Read the model definition and answer for the solid it produces. Units are mm, in the model's axes. A direction names the side the tool comes from. Coordinates: 2 decimals unless noted, no trailing zeros. Write each loop counter-clockwise with the first axis right and the second up, starting at its lowest first coordinate (ties: lowest second). Pieces come first, ordered by that corner, then holes. Notation, with made-up numbers: M 42,-27.5 L 75,-27.5 A17 cw 75,-22.5 Z; hole C -3.75,-11 d7. An arc over 180 degrees is marked long. Write item = value, one per line.
from build123d import *

# Parameters (mm, degrees)
SKETCH_1_W      = 40
SKETCH_1_H      = 53.5
SKETCH_1_R      = 6.25
SKETCH_1_R_2    = 2
SKETCH_1_W_2    = 3.5
SKETCH_1_H_2    = 1.5
SKETCH_1_W_3    = 1.5
SKETCH_1_H_3    = 3.5
EXTRUDE_1_DEPTH = 5
FILLET_1_R      = 3


with BuildPart() as part:
    # ｽｹｯﾁ1 → ﾎﾞｽ - 押し出し1 (new body)
    with BuildSketch(Plane.XY):
        with Locations((20, 26.75)):
            Rectangle(SKETCH_1_W, SKETCH_1_H)
        with Locations((20, 26.75)):
            Circle(SKETCH_1_R, mode=Mode.SUBTRACT)
        with Locations((35, 5)):
            Circle(SKETCH_1_R_2, mode=Mode.SUBTRACT)
        with Locations(Location((5, 5, 0), (0, 0, 180))):
            Circle(SKETCH_1_R_2, mode=Mode.SUBTRACT)
        with Locations((20, 35.75)):
            Rectangle(SKETCH_1_W_2, SKETCH_1_H_2, mode=Mode.SUBTRACT)
        with Locations((11, 26.75)):
            Rectangle(SKETCH_1_W_3, SKETCH_1_H_3, mode=Mode.SUBTRACT)
    extrude(amount=EXTRUDE_1_DEPTH)

    # ﾌｨﾚｯﾄ1
    fillet_1_edges = [part.edges().sort_by_distance(p)[0] for p in [
        (0, 53.5, 2.5),
        (40, 53.5, 2.5),
        (40, 0, 2.5),
        (0, 0, 2.5),
    ]]
    fillet(fillet_1_edges, radius=FILLET_1_R)


solid = part.part
Item 1: Find section A-A (x = 35). Determine the outline of the cut face in (y, z), and give its area (4 significant figures).
Worked answers:
outline = M 0,0 L 3,0 L 3,5 L 0,5 Z; M 7,0 L 53.5,0 L 53.5,5 L 7,5 Z
area = 247.5 mm²
Item 2: Find section B-B (y = 5). Determine the outline of the cut face in (x, z).
Worked answers:
outline = M 0,0 L 3,0 L 3,5 L 0,5 Z; M 7,0 L 33,0 L 33,5 L 7,5 Z; M 37,0 L 40,0 L 40,5 L 37,5 Z
Item 3: Find section D-D (z = 3.4). Determine the outline of the cut face in (x, y), and give its area (3 significant figures).
Worked answers:
outline = M 0,3 A3 ccw 3,0 L 37,0 A3 ccw 40,3 L 40,50.5 A3 ccw 37,53.5 L 3,53.5 A3 ccw 0,50.5 Z; hole C 5,5 d4; hole M 10.25,25 L 11.75,25 L 11.75,28.5 L 10.25,28.5 Z; hole C 20,26.75 d12.5; hole M 18.25,35 L 21.75,35 L 21.75,36.5 L 18.25,36.5 Z; hole C 35,5 d4
area = 1,970 mm²
Item 4: Consider line 1 along Y through (x, z) = (20, 1.55); line 2 along X through (y, z) = (26.5, 0.9) (3 decimals); line 3 along Y through (x, z) = (35, 2.55). Determine where each line is inside the solid, lowest interval first. Write a range as from..to.
Worked answers:
line_1 = 0..20.5, 33..35, 36.5..53.5
line_2 = 0..10.25, 11.75..13.755, 26.245..40
line_3 = 0..3, 7..53.5
Item 5: Find section C-C (x = 20). Determine the outline of the cut face in (y, z).
Worked answers:
outline = M 0,0 L 20.5,0 L 20.5,5 L 0,5 Z; M 33,0 L 35,0 L 35,5 L 33,5 Z; M 36.5,0 L 53.5,0 L 53.5,5 L 36.5,5 Z
Item 6: Which of the six approach directions +Z, -Z, +X, -X, +Y, -Y give full straight-line access (tool end or side, diameter ignored) to faces 5 (the face through (21.75, 36, 2)), 6 (the face through (0.86, 0.9, 2.54))?
Worked answers:
face_5 = +Z, -Z
face_6 = +Z, -Z, -X, -Y
Item 7: For a pull along Y with two mould halves and no side action, classify faces 1 (the face through (39.1, 0.86, 2.54)), 2 (the face through (11, 28.5, 2)), 3 (the face through (40, 26, 2)), 4 (the face through (39.1, 52.64, 2.54)) as released by +Y, released by -Y, zero draft, split by the parting line, or undercut.
Worked answers:
face_1 = released by -Y
face_2 = undercut
face_3 = zero draft
face_4 = released by +Y
